Design review of the part built by this model. Coordinates are the model's own, in mm. Face numbers are marked on the shaded views. A direction names the side the tool comes from. Coordinates: 2 decimals unless noted, no trailing zeros. Order: outer loops, then holes, each group sorted by start corner. A loop starts at its lowest first (then second) coordinate and runs counter-clockwise, first axis right, second up.
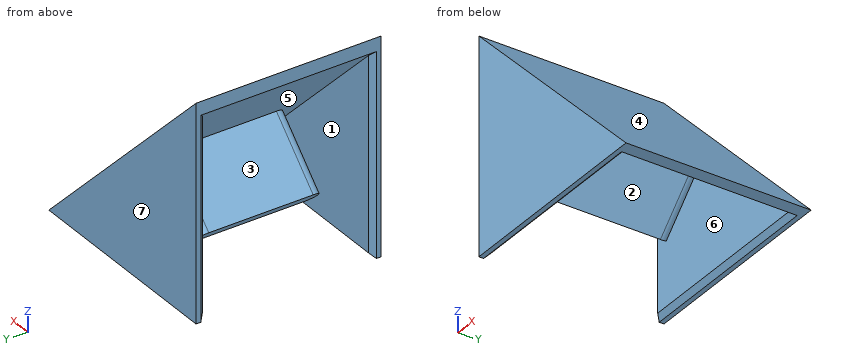
from build123d import *

# Parameters (mm, degrees)
F1_DEPTH = 19.5
F2_T     = -1
F4_DEPTH = 8
F5_SIZE  = 0.5


with BuildPart() as f1:
    # F0 (on Front) → F1 (new body)
    with BuildSketch(Plane.XZ):
        Polygon((-11.313708499, 11.313708499), (-11.313708499, -11.313708499), (11.313708499, -11.313708499), align=None)
    extrude(amount=F1_DEPTH)

    # F2
    f2_openings = [f1.faces().sort_by_distance(p)[0] for p in [
        (0, -9.75, -11.313708),
        (-11.313708, -9.75, 0),
    ]]
    offset(amount=F2_T, openings=f2_openings)

    # F3 (on face) → F4 (join)
    with BuildSketch(Plane(origin=(-0.7071067812, 0, -0.7071067812), x_dir=(0, -1, 0), z_dir=(-0.7071067812, 0, -0.7071067812))):
        with BuildLine():
            Line((15.25, 1), (4.25, 1))
            ThreePointArc((4.25, 1), (3.5428932188, 0.7071067812), (3.25, 0))
            ThreePointArc((3.25, 0), (3.5428932188, -0.7071067812), (4.25, -1))
            Line((4.25, -1), (15.25, -1))
            ThreePointArc((15.25, -1), (15.9571067812, -0.7071067812), (16.25, 0))
            ThreePointArc((16.25, 0), (15.9571067812, 0.7071067812), (15.25, 1))
        make_face()
    extrude(amount=F4_DEPTH)

    # F5
    f5_edges = [f1.edges().sort_by_distance(p)[0] for p in [
        (-0.707107, -1, -11.313708),
        (-11.313708, -1, -0.707107),
        (-11.313708, -18.5, -0.707107),
        (-0.707107, -18.5, -11.313708),
    ]]
    chamfer(f5_edges, length=F5_SIZE)


solid = f1.part
1. Add section D-D (y = -18). Give the boundary of the cut face in (x, z), and give its area (3 significant figures).
2. Mouldability with a two-part tool opening along Z and no side actions: class the marked faces 1, 2, 3 and 4 as pulls with the +Z half, pulls with the -Z half, needs draft (parallel to the pull), parting line crosses it, or undercut.
3. For the marked faces 5, 6 and 7, list the 3-axis set-ups (+Z, -Z, +X, -X, +Y, -Y) from which the entire face can be reached by the end or side of a thin tool; tool diameter is ignored.
4. Add section C-C (z = -9.25). Give the boundary of the cut face in (x, y).
5. Add section B-B (x = 1.5). Give the boundary of the cut face in (y, z).
6. Add section A-A (y = -6.5). Give the boundary of the cut face in (x, z), and give its area (3 significant figures).
7. To check wall thickness, follow line 1 (Y direction, x = -9.75, z = -3.25); line 2 (Z direction, x = -4, y = -10.5); line 3 (X direction, y = -6.25, z = -1.75). State the ranges of each line that lie inside material, in increasing order.
8. Insertion check: pin 1 (10 mm diameter, centred on y = -11, z = -2, fed in from +X); pin 2 (1 mm diameter, centred on x = 7, y = -5.5, fed in from -Z); pin 3 (6 mm diameter, centred on x = 5, y = -10.5, fed in from -Z). Each pin has a flat end and moves straight along its axis. Give the tip position at first contact, or say it passes through.
Solution:
1. outline: (-11.31, 9.9) - (9.9, -11.31) - (11.31, -11.31) - (-11.31, 11.31) - close
1. area: 31.0 mm2
2. face 1: needs draft
2. face 2: pulls with the -Z half
2. face 3: undercut
2. face 4: pulls with the +Z half
3. face 5: none
3. face 6: -Z, -X
3. face 7: +Z, -Z, +X, -X, +Y
4. outline: (-11.31, -19.5) - (9.25, -19.5) - (9.25, 0) - (-11.31, 0) - (-11.31, -0.5) - (-10.81, -1) - (7.84, -1) - (7.84, -18.5) - (-10.81, -18.5) - (-11.31, -19) - close
5. outline: (-19.5, -11.31) - (-19, -11.31) - (-18.5, -10.81) - (-18.5, -2.91) - (-1, -2.91) - (-1, -10.81) - (-0.5, -11.31) - (0, -11.31) - (0, -1.5) - (-19.5, -1.5) - close
6. outline: (-11.31, 9.9) - (-1.41, 0) - (-7.07, -5.66) - (-5.66, -7.07) - (0, -1.41) - (9.9, -11.31) - (11.31, -11.31) - (-11.31, 11.31) - close
6. area: 47.0 mm2
7. line 1: y = -19.5 to -18.5, -1 to 0
7. line 2: z = -5.41 to -2.59, 2.59 to 4
7. line 3: x = -3.16 to -0.34, 0.34 to 1.75
8. pin 1: stops at x = 7
8. pin 2: stops at z = -8.91
8. pin 3: stops at z = -9.41
